Part model, mm, in its own coordinate system. Coordinates: 2 decimals unless noted, no trailing zeros.
from build123d import *

# Parameters (mm, degrees)
SKIZZE1_W                       = 500
SKIZZE1_H                       = 360
AUFSATZ_LINEAR_AUSTRAGEN1_DEPTH = 20
FASE1_SIZE                      = 10
SKIZZE2_R                       = 2.5
SCHNITT_LINEAR_AUSTRAGEN1_DEPTH = 309.706980809


with BuildPart() as part:
    # Skizze1 → Aufsatz-Linear austragen1 (new body)
    with BuildSketch(Plane(origin=(0, 0, 0), x_dir=(1, 0, 0), z_dir=(0, 1, 0))):
        Rectangle(SKIZZE1_W, SKIZZE1_H)
    extrude(amount=AUFSATZ_LINEAR_AUSTRAGEN1_DEPTH)

    # Fase1
    fase1_edges = [part.edges().sort_by_distance(p)[0] for p in [
        (-250, 20, 0),
        (0, 20, 180),
        (250, 20, 0),
        (0, 20, -180),
    ]]
    chamfer(fase1_edges, length=FASE1_SIZE)

    # Skizze2 → Schnitt-Linear austragen1 (cut, through all)
    with BuildSketch(Plane(origin=(0, 20, 0), x_dir=(1, 0, 0), z_dir=(0, 1, 0))):
        with Locations(Location((-227.5, -157.5, 0), (0, 0, 270))):
            Circle(SKIZZE2_R)
        with Locations(Location((-142.5, -157.5, 0), (0, 0, 270))):
            Circle(SKIZZE2_R)
        with Locations(Location((102.5, -157.5, 0), (0, 0, 270))):
            Circle(SKIZZE2_R)
        with Locations(Location((227.5, -157.5, 0), (0, 0, 270))):
            Circle(SKIZZE2_R)
        with Locations(Location((-227.5, 157.5, 0), (0, 0, 270))):
            Circle(SKIZZE2_R)
        with Locations(Location((-142.5, 157.5, 0), (0, 0, 270))):
            Circle(SKIZZE2_R)
        with Locations(Location((102.5, 157.5, 0), (0, 0, 270))):
            Circle(SKIZZE2_R)
        with Locations(Location((227.5, 157.5, 0), (0, 0, 270))):
            Circle(SKIZZE2_R)
    extrude(amount=-SCHNITT_LINEAR_AUSTRAGEN1_DEPTH, mode=Mode.SUBTRACT)


solid = part.part
Q1. Cut at A-A on y = 15.75. Count the separate pieces of the cut face and the enclosed holes in it, and give its area (3 significant figures).
Results list:
separate pieces: 1
enclosed holes: 8
area: 170,000 mm2
Q2. Pin check, flat tips, straight feed: pin 1 Ø4 at (x, y) = (-29.5, 12.5) entering from -Z; pin 2 Ø5 at (y, z) = (15.5, -117) entering from +X; pin 3 Ø4.5 at (x, z) = (-227.5, 157.5) entering from -Y. Stop position of each tip, or through.
Results list:
pin 1: stops at z = -179.5
pin 2: stops at x = 247
pin 3: passes through
Q3. Wall check: line 1 along Z through (x, y) = (-227.5, 5); line 2 along Z through (x, y) = (227, 2.25); line 3 along X through (y, z) = (8.25, -157.5). Give the ranges that are in metal, low to high.
Results list:
line 1: z = -180 to -160, -155 to 155, 160 to 180
line 2: z = -180 to -159.95, -155.05 to 155.05, 159.95 to 180
line 3: x = -250 to -230, -225 to -145, -140 to 100, 105 to 225, 230 to 250
